The model under review builds one solid part; all positions refer to its coordinate system, in mm. A direction names the side the tool comes from. Coordinates: 2 decimals unless noted, no trailing zeros. Order: outer loops, then holes, each group sorted by start corner. A loop starts at its lowest first (then second) coordinate and runs counter-clockwise, first axis right, second up. Notation, with made-up numbers: M 53.25,-28.75 L 104.25,-28.75 A25 ccw 104.25,2.25 Z; hole C 47.25,-35.5 d5. An arc over 180 degrees is marked long. Answer as CSV lines item,"result". Start each with the question number.
Q1. Wall thickness on L1, parallel to Y at x = 0, z = 17.5; L2, parallel to Y at x = -38, z = 23.2; L3, parallel to X at y = 16.75, z = 23.75: over which ranges is each line inside the solid? List them lowest first. Write a range as [from, to].
Q2. For P1, Ø3.5, axis at y = 10, z = 24, coming from the -X side; P2, Ø0.9, axis at y = 5.5, z = 23.5, coming from the +X side; P3, Ø1, axis at x = -38, y = 16.5, coming from the +Z side, all flat-tipped, find the tip position at first contact; note any pin that passes through.
Q3. Consider section A-A on y = -41. Write out the cut boundary in (x, z).
Q4. Consider section B-B on x = 0. Write out the cut boundary in (y, z).
Q5. Consider section C-C on y = 35.5. Write out the cut boundary in (x, z).
Q6. The part is to be moulded in two halves that separate along X. For faces 1 (the face through (-1, 20, 23)), 2 (the face through (-44, 0, 23)), 3 (the face through (-0.38, -42.71, 10.85)), say which applies: +X half, -X half, draft (parallel to the pull), parting line (faces both ways), or undercut.
Q7. Machinability: for faces 4 (the face through (-1, -20, 23)), 5 (the face through (44, 0, 23)), 6 (the face through (-1, -60, 11)), which of the approach directions +Z, -Z, +X, -X, +Y, -Y give a long, thin tool a straight path to every point of the face, cutting with its end or side? Answer none if there is none.
from build123d import *

# Parameters (mm, degrees)
SKETCH1_W           = 90
SKETCH1_H           = 120
SKETCH1_R           = 1.75
BOSS_EXTRUDE1_DEPTH = 22
SKETCH3_W           = 88
SKETCH3_H           = 40
SKETCH3_R           = 1
BOSS_EXTRUDE2_DEPTH = 25


with BuildPart() as part:
    # Sketch1 → Boss-Extrude1 (new body)
    with BuildSketch(Plane.XY):
        Rectangle(SKETCH1_W, SKETCH1_H)
        with Locations((0, 41)):
            Circle(SKETCH1_R, mode=Mode.SUBTRACT)
        with Locations((0, -41)):
            Circle(SKETCH1_R, mode=Mode.SUBTRACT)
    extrude(amount=BOSS_EXTRUDE1_DEPTH)

    # Sketch3 → Boss-Extrude2 (add)
    with BuildSketch(Plane.XY):
        Rectangle(SKETCH3_W, SKETCH3_H)
        with Locations((-38, 16.75)):
            Circle(SKETCH3_R, mode=Mode.SUBTRACT)
        with Locations((38, -16.75)):
            Circle(SKETCH3_R, mode=Mode.SUBTRACT)
    extrude(amount=BOSS_EXTRUDE2_DEPTH)


solid = part.part
Evaluation:
1,L1,"y = [-60, -42.75], [-39.25, 39.25], [42.75, 60]"
1,L2,"y = [-20, 15.75], [17.75, 20]"
1,L3,"x = [-44, -39], [-37, 44]"
2,P1,"stops at x = -44"
2,P2,"stops at x = 44"
2,P3,"stops at z = 22"
3,outline,"M -45,0 L -1.75,0 L -1.75,22 L -45,22 Z; M 1.75,0 L 45,0 L 45,22 L 1.75,22 Z"
4,outline,"M -60,0 L -42.75,0 L -42.75,22 L -60,22 Z; M -39.25,0 L 39.25,0 L 39.25,22 L 20,22 L 20,25 L -20,25 L -20,22 L -39.25,22 Z; M 42.75,0 L 60,0 L 60,22 L 42.75,22 Z"
5,outline,"M -45,0 L 45,0 L 45,22 L -45,22 Z"
6,face 1,"draft"
6,face 2,"-X half"
6,face 3,"undercut"
7,face 4,"+Z, +X, -X, -Y"
7,face 5,"+Z, +X, +Y, -Y"
7,face 6,"+Z, -Z, +X, -X, -Y"
